Design review of the part built by this model. Coordinates are the model's own, in mm. A direction names the side the tool comes from. Coordinates: 2 decimals unless noted, no trailing zeros. Order: outer loops, then holes, each group sorted by start corner. A loop starts at its lowest first (then second) coordinate and runs counter-clockwise, first axis right, second up.
from build123d import *

# Parameters (mm, degrees)
SKETCH2_W           = 20
SKETCH2_H           = 3
SKETCH2_W_2         = 3
SKETCH2_H_2         = 15
BOSS_EXTRUDE1_DEPTH = 3


with BuildPart() as part:
    # Sketch2 → Boss-Extrude1 (new body)
    with BuildSketch(Plane.XY):
        Polygon((45, -40), (56, -40), (56, -27.5), (56, -12.5), (56, 2.5), (-56, 2.5), (-56, -12.5), (-56, -27.5), (-56, -40), (-45, -40), (-25, -40), (-10, -40), (10, -40), (25, -40), align=None)
        with Locations((35, -41.5)):
            Rectangle(SKETCH2_W, SKETCH2_H)
        with Locations((57.5, -20)):
            Rectangle(SKETCH2_W_2, SKETCH2_H_2)
        with Locations((0, -41.5)):
            Rectangle(SKETCH2_W, SKETCH2_H)
        Polygon((-56, 2.5), (56, 2.5), (56, 17.5), (56, 40), (-56, 40), (-56, 17.5), align=None)
        with Locations((57.5, 10)):
            Rectangle(SKETCH2_W_2, SKETCH2_H_2)
        with Locations((-57.5, 10)):
            Rectangle(SKETCH2_W_2, SKETCH2_H_2)
        with Locations((-35, -41.5)):
            Rectangle(SKETCH2_W, SKETCH2_H)
        with Locations((-57.5, -20)):
            Rectangle(SKETCH2_W_2, SKETCH2_H_2)
    extrude(amount=BOSS_EXTRUDE1_DEPTH)


solid = part.part
1. To check wall thickness, follow line 1 (X direction, y = -2, z = 2.3); line 2 (Y direction, x = -49.5, z = 0.25). State the ranges of each line that lie inside material, in increasing order.
2. Add section C-C (y = 23). Give the boundary of the cut face in (x, z), and give its area (3 significant figures).
3. Add section B-B (x = 12.5). Give the boundary of the cut face in (y, z), and give its area (3 significant figures).
4. Insertion check: pin 1 (1.5 mm diameter, centred on x = -58, z = 1, fed in from -Y); pin 2 (1.5 mm diameter, centred on y = -41.5, z = 2, fed in from +X); pin 3 (0.9 mm diameter, centred on y = -41, z = 1.5, fed in from -X); pin 4 (12 mm diameter, centred on x = -45, y = -16, fed in from -Z). Each pin has a flat end and moves straight along its axis. Give the tip position at first contact, or say it passes through.
5. Mouldability with a two-part tool opening along Y and no side actions: class faces 6 (the flat face through (56, -5, 1)), 7 (the flat face through (17, -40, 1)), 8 (the flat face through (-58, 2.5, 1)), 9 (the flat face through (45, -42, 1)) as pulls with the +Y half, pulls with the -Y half, needs draft (parallel to the pull), parting line crosses it, or undercut.
6. For faces 1 (the flat face through (-58, -27.5, 1)), 2 (the flat face through (-58, 17.5, 1)), 3 (the flat face through (25, -42, 1)), 4 (the flat face through (57, 17.5, 1)), 5 (the flat face through (50, -40, 1)), list the 3-axis set-ups (+Z, -Z, +X, -X, +Y, -Y) from which the entire face can be reached by the end or side of a thin tool; tool diameter is ignored.
Solution:
1. line 1: x = -56 to 56
1. line 2: y = -40 to 40
2. outline: (-56, 0) - (56, 0) - (56, 3) - (-56, 3) - close
2. area: 336 mm2
3. outline: (-40, 0) - (40, 0) - (40, 3) - (-40, 3) - close
3. area: 240 mm2
4. pin 1: stops at y = -27.5
4. pin 2: stops at x = 45
4. pin 3: stops at x = -45
4. pin 4: stops at z = 0
5. face 6: undercut
5. face 7: pulls with the -Y half
5. face 8: undercut
5. face 9: needs draft
6. face 1: +Z, -Z, -X, -Y
6. face 2: +Z, -Z, -X, +Y
6. face 3: +Z, -Z, -Y
6. face 4: +Z, -Z, +X, +Y
6. face 5: +Z, -Z, +X, -Y
